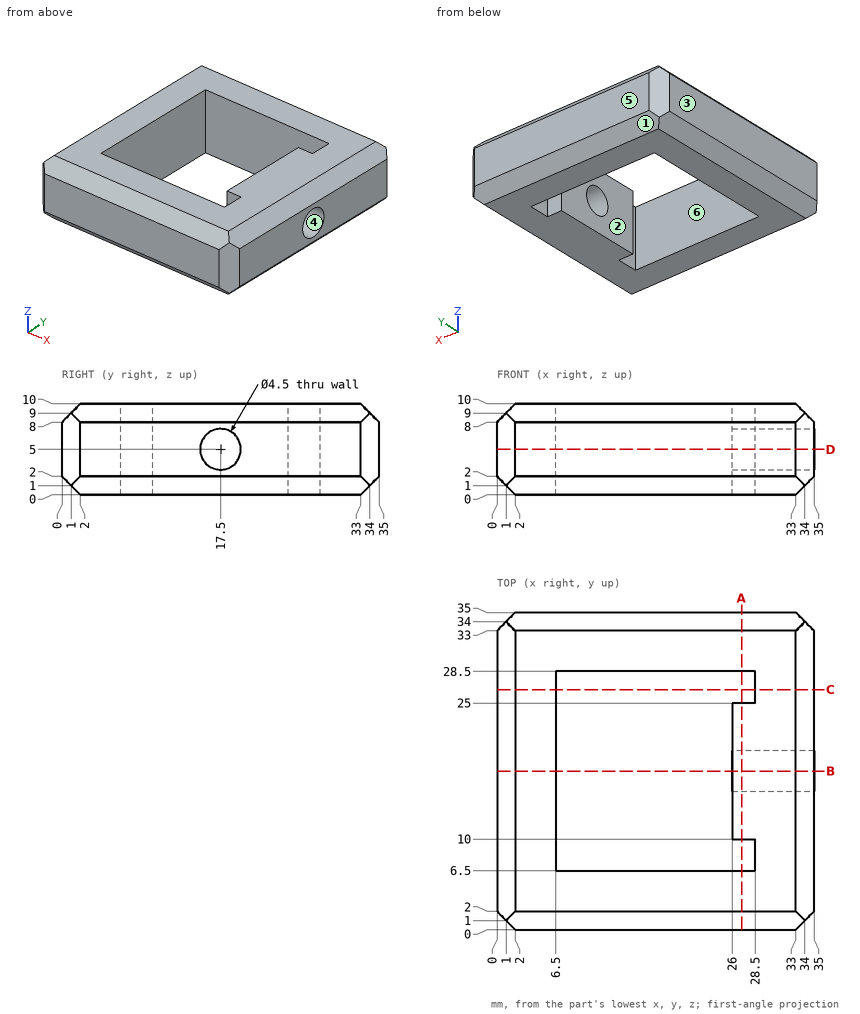
Answer from the drawing. Dimensions are ordinates in mm from the lowest x, y and z of the part. A direction names the side the tool comes from. Round coordinates to 2 decimals unless told otherwise and drop trailing zeros. Order: outer loops, then holes, each group sorted by start corner. A loop starts at its lowest first (then second) coordinate and runs counter-clockwise, first axis right, second up.
1) The part is cut by section D-D on z = 5. Write down the section's boundary in (x, y), plus the area to 3 significant figures.
2) The part is cut by section A-A on x = 27. Write down the section's boundary in (y, z).
3) The part is cut by section C-C on y = 26.5. Write down the section's boundary in (x, z).
4) Straight lines are drawn through the part: L1, parallel to Z at x = 31, y = 17.5; L2, parallel to X at y = 24, z = 3.75; L3, parallel to X at y = 26, z = 2.5. For each, find the intervals that lie inside material, in ascending order.
5) The mould has two halves that part along X. Classify the marked faces 1, 2 and 3: released by +X, released by -X, zero draft, split by the parting line, or undercut.
6) For the marked faces 4, 5 and 6, determine the directions among +Z, -Z, +X, -X, +Y, -Y from which every point of the face is accessible in a straight line to the end or side of a thin tool.
7) A flat-ended cylindrical pin translates along its axis: pin 1 (10 mm diameter, centred on x = 16, y = 21.5, fed in from -Z). Find the tip coordinate at first contact, or state that the pin passes through.
8) The part is cut by section B-B on y = 17.5. Write down the section's boundary in (x, z).
Resolved:
1. outline: (0, 2) - (2, 0) - (33, 0) - (35, 2) - (35, 15.25) - (26, 15.25) - (26, 10) - (28.5, 10) - (28.5, 6.5) - (6.5, 6.5) - (6.5, 28.5) - (28.5, 28.5) - (28.5, 25) - (26, 25) - (26, 19.75) - (35, 19.75) - (35, 33) - (33, 35) - (2, 35) - (0, 33) - close
1. area: 730 mm2
2. outline: (0, 2) - (2, 0) - (6.5, 0) - (6.5, 10) - (2, 10) - (0, 8) - close; (10, 0) - (25, 0) - (25, 10) - (10, 10) - close; (28.5, 0) - (33, 0) - (35, 2) - (35, 8) - (33, 10) - (28.5, 10) - close; hole circle Ø4.5 at (17.5, 5)
3. outline: (0, 2) - (2, 0) - (6.5, 0) - (6.5, 10) - (2, 10) - (0, 8) - close; (28.5, 0) - (33, 0) - (35, 2) - (35, 8) - (33, 10) - (28.5, 10) - close
4. L1: z = 0 to 2.75, 7.25 to 10
4. L2: x = 0 to 6.5, 26 to 35
4. L3: x = 0 to 6.5, 28.5 to 35
5. face 1: zero draft
5. face 2: undercut
5. face 3: released by -X
6. face 4: +X
6. face 5: +Z, -Z, +X, -X, +Y
6. face 6: +Z, -Z
7. pin 1: passes through
8. outline: (0, 2) - (2, 0) - (6.5, 0) - (6.5, 10) - (2, 10) - (0, 8) - close; (26, 0) - (33, 0) - (35, 2) - (35, 2.75) - (26, 2.75) - close; (26, 7.25) - (35, 7.25) - (35, 8) - (33, 10) - (26, 10) - close
